```python
from build123d import *

# Parameters (mm, degrees)
BOSS_EXTRUDE1_DEPTH     = 92.5
SKETCH2_W               = 80
SKETCH2_H               = 170
CUT_EXTRUDE1_DEPTH      = 2.5
FILLET1_R               = 10
CUT_EXTRUDE2_DEPTH      = 158.5
CUT_EXTRUDE2_DEPTH_BACK = 158.5
SKETCH3_R               = 1.5


with BuildPart() as part:
    # Sketch1 → Boss-Extrude1 (new, symmetric)
    with BuildSketch(Plane.XY):
        with BuildLine():
            Line((-60, 55), (0, 55))
            Line((0, 55), (0, 52.5))
            Line((0, 52.5), (-60, 52.5))
            ThreePointArc((-60, 52.5), (-112.5, 0), (-60, -52.5))
            Line((-60, -52.5), (0, -52.5))
            Line((0, -52.5), (0, -55))
            Line((0, -55), (-60, -55))
            ThreePointArc((-60, -55), (-115, 0), (-60, 55))
        make_face()
    extrude(amount=BOSS_EXTRUDE1_DEPTH, both=True)

    # Sketch2 → Cut-Extrude1 (cut)
    with BuildSketch(Plane.XZ.offset(55)):
        Rectangle(SKETCH2_W, SKETCH2_H)
    extrude(amount=-CUT_EXTRUDE1_DEPTH, mode=Mode.SUBTRACT)

    # Fillet1
    fillet1_edges = [part.edges().sort_by_distance(p)[0] for p in [
        (-40, -53.75, 85),
        (-40, -53.75, -85),
    ]]
    fillet(fillet1_edges, radius=FILLET1_R)

    # Sketch3 → Cut-Extrude2 (cut, two sides: drawn at the far end of the back side and taken through both)
    with BuildSketch(Plane(origin=(0, 0, 0), x_dir=(1, 0, 0), z_dir=(0, 1, 0)).offset(-CUT_EXTRUDE2_DEPTH_BACK)):
        with Locations(Location((-55, 88.75, 0), (0, 0, 270))):
            Circle(SKETCH3_R)
        with Locations(Location((-33, 88.75, 0), (0, 0, 270))):
            Circle(SKETCH3_R)
        with Locations(Location((-11, 88.75, 0), (0, 0, 270))):
            Circle(SKETCH3_R)
        with Locations(Location((-11, -88.75, 0), (0, 0, 270))):
            Circle(SKETCH3_R)
        with Locations(Location((-33, -88.75, 0), (0, 0, 270))):
            Circle(SKETCH3_R)
        with Locations(Location((-55, -88.75, 0), (0, 0, 270))):
            Circle(SKETCH3_R)
    extrude(amount=CUT_EXTRUDE2_DEPTH + CUT_EXTRUDE2_DEPTH_BACK, mode=Mode.SUBTRACT)


solid = part.part
```
Can you work these out from the model? Positions are in its coordinate system, mm. A direction names the side the tool comes from. Round coordinates to 2 decimals unless told otherwise and drop trailing zeros. Loops run counter-clockwise (first coordinate to the right, second up) from the corner with the lowest first, then second, coordinate; pieces in that order, holes last.
Item 1: Which directions (+Z, -Z, +X, -X, +Y, -Y) give clear straight access to the entire face, cutting with the end or side of a thin tool? Please do faces 1 (the cylindrical face through (-37.15, -53.73, 81.99)), 2 (the flat face through (-104, 29, 92.5)).
Item 2: Will these pins go through, and if not, where does the flat tip stop? pin 1 Ø3 at (x, z) = (-87.5, 40) entering from -Y; pin 2 Ø3.5 at (x, z) = (-55, 88.75) entering from -Y; pin 3 Ø0.8 at (y, z) = (-54, -27.5) entering from +X; pin 4 Ø8 at (x, z) = (-16, -20) entering from -Y.
Item 3: Suppose I cut it at C-C, the plane y = 0. Write out the boundary of the cut face in (x, z), then the cut area to 4 significant figures.
Item 4: Suppose I cut it at B-B, the plane z = 1.5. Write out the boundary of the cut face in (x, y).
Item 5: Suppose I cut it at D-D, the plane x = -105. Write out the boundary of the cut face in (y, z), then the cut area to 3 significant figures.
Item 6: If we mould it in two halves opening along Y, with no side actions, what happens to faces 3 (the flat face through (-43, -52.5, 0)), 4 (the cylindrical face through (-36.99, -53.73, -82.15)), 5 (the flat face through (-30, 52.5, 1)), 6 (the cylindrical face through (-114.987, -1.209, 1.295))? For each: +Y half, -Y half, draft (parallel to the pull), parting line (faces both ways), or undercut.
Item 7: Please list where these lines run through material, in increasing order: L1, parallel to Z at x = -33, y = 53; L2, parallel to Z at x = -11, y = -53; L3, parallel to Y at x = -47, z = 76.
Item 8: Suppose I cut it at A-A, the plane x = -46.5. Write out the boundary of the cut face in (y, z).
Reported:
1. face 1: +X, -Y
1. face 2: +Z, +X, -X, +Y, -Y
2. pin 1: stops at y = -48.47
2. pin 2: stops at y = -55
2. pin 3: stops at x = -40
2. pin 4: stops at y = 52.5
3. outline: (-115, -92.5) - (-112.5, -92.5) - (-112.5, 92.5) - (-115, 92.5) - close
3. area: 462.5 mm2
4. outline: (-60, -55) - (-40, -55) - (-40, -52.5) - (-60, -52.5) arc R52.5 cw to (-60, 52.5) - (0, 52.5) - (0, 55) - (-60, 55) arc R55 ccw to start
5. outline: (-31.62, -92.5) - (-27.04, -92.5) - (-27.04, 92.5) - (-31.62, 92.5) - close; (27.04, -92.5) - (31.62, -92.5) - (31.62, 92.5) - (27.04, 92.5) - close
5. area: 1,700 mm2
6. face 3: undercut
6. face 4: draft
6. face 5: undercut
6. face 6: parting line
7. L1: z = -92.5 to -90.25, -87.25 to 87.25, 90.25 to 92.5
7. L2: z = -92.5 to -90.25, -87.25 to -85, 85 to 87.25, 90.25 to 92.5
7. L3: y = -55 to -52.5, 52.5 to 55
8. outline: (-55, -92.5) - (-52.5, -92.5) - (-52.5, 92.5) - (-55, 92.5) - close; (52.5, -92.5) - (55, -92.5) - (55, 92.5) - (52.5, 92.5) - close
